The listing builds one solid part. Answer for the finished solid, in the listing's coordinates (mm). A direction names the side the tool comes from. Coordinates: 2 decimals unless noted, no trailing zeros. Write each loop counter-clockwise with the first axis right and the second up, starting at its lowest first coordinate (ties: lowest second). Pieces come first, ordered by that corner, then holes. Notation, with made-up numbers: M 53,53 L 81,53 A36 cw 81,92 Z; hole C 32.25,56 d1. An arc over 180 degrees is marked long. Answer as CSV lines item,"result".
```python
from build123d import *

# Parameters (mm, degrees)
SKETCH1_R           = 37.5
BOSS_EXTRUDE1_DEPTH = 10
BOSS_EXTRUDE2_START = 10
BOSS_EXTRUDE2_DEPTH = 10
SKETCH3_R           = 2.55
CUT_EXTRUDE1_DEPTH  = 10


with BuildPart() as part:
    # Sketch1 → Boss-Extrude1 (new body)
    with BuildSketch(Plane(origin=(0, 0, 0), x_dir=(1, 0, 0), z_dir=(0, 1, 0))):
        with Locations(Location((11.945516858, 0, 0), (0, 0, 270))):
            Circle(SKETCH1_R)
    extrude(amount=BOSS_EXTRUDE1_DEPTH)

    # Sketch2 → Boss-Extrude2 (add)
    with BuildSketch(Plane(origin=(0, 0, 0), x_dir=(1, 0, 0), z_dir=(0, 1, 0)).offset(BOSS_EXTRUDE2_START)):
        with BuildLine():
            Line((-6.304483142, 19.484324941), (30.195516858, 19.484324941))
            ThreePointArc((30.195516858, 19.484324941), (37.26658467, 16.555392753), (40.195516858, 9.484324941))
            Line((40.195516858, 9.484324941), (40.195516858, -9.205373472))
            ThreePointArc((40.195516858, -9.205373472), (37.270385296, -16.272638614), (30.20626954, -19.205367691))
            Line((30.20626954, -19.205367691), (-6.29373046, -19.244615001))
            ThreePointArc((-6.29373046, -19.244615001), (-13.371748284, -16.319489219), (-16.304483142, -9.244620782))
            Line((-16.304483142, -9.244620782), (-16.304483142, 9.484324941))
            ThreePointArc((-16.304483142, 9.484324941), (-13.375550954, 16.555392753), (-6.304483142, 19.484324941))
        make_face()
        Polygon((-11.304483142, -14.250000016), (35.195516858, -14.200000018), (35.195516858, 14.484324941), (-11.304483142, 14.484324941), align=None, mode=Mode.SUBTRACT)
    extrude(amount=BOSS_EXTRUDE2_DEPTH)

    # Sketch3 → Cut-Extrude1 (cut)
    with BuildSketch(Plane(origin=(0, 10, 0), x_dir=(1, 0, 0), z_dir=(0, 1, 0))):
        with Locations(Location((-21.054483142, -5, 0), (0, 0, 270))):
            Circle(SKETCH3_R)
        with Locations(Location((-21.054483142, 5, 0), (0, 0, 90))):
            Circle(SKETCH3_R)
        with Locations(Location((44.945516858, -5, 0), (0, 0, 90))):
            Circle(SKETCH3_R)
        with Locations(Location((44.945516858, 5, 0), (0, 0, 270))):
            Circle(SKETCH3_R)
    extrude(amount=-CUT_EXTRUDE1_DEPTH, mode=Mode.SUBTRACT)


solid = part.part
```
Q1. For faces 5 (the flat face through (-11.304, 15, 0)), 6 (the cylindrical face through (-13.45, 14.93, -16.48)), 7 (the cylindrical face through (37.19, 14.93, -16.63)), determine the directions among +Z, -Z, +X, -X, +Y, -Y from which every point of the face is accessible in a straight line to the end or side of a thin tool.
Output:
face 5,"+Y"
face 6,"-Z, -X, +Y"
face 7,"-Z, +X, +Y"
Q2. Find section B-B (z = -5). Give the vertices of the cut face in (x, y).
Output:
outline,"M -25.22,0 L -23.6,0 L -23.6,10 L -25.22,10 Z; M -18.5,0 L 42.4,0 L 42.4,10 L 40.2,10 L 40.2,20 L 35.2,20 L 35.2,10 L -11.3,10 L -11.3,20 L -16.3,20 L -16.3,10 L -18.5,10 Z; M 47.5,0 L 49.11,0 L 49.11,10 L 47.5,10 Z"
Q3. Find section D-D (x = 16). Give the vertices of the cut face in (y, z), and give its area (3 significant figures).
Output:
outline,"M 0,-37.28 L 10,-37.28 L 10,-19.48 L 20,-19.48 L 20,-14.48 L 10,-14.48 L 10,14.22 L 20,14.22 L 20,19.22 L 10,19.22 L 10,37.28 L 0,37.28 Z"
area,"846 mm2"
Q4. Straight lines are drawn through the part: line 1 (Z direction, x = -21.5, y = 2.75); line 2 (X direction, y = 4.25, z = -5); line 3 (Z direction, x = 2, y = 10.75). For each, find the intervals that lie inside material, in ascending order.
Output:
line 1,"-16.96 to -7.51, -2.49 to 2.49, 7.51 to 16.96"
line 2,"-25.22 to -23.6, -18.5 to 42.4, 47.5 to 49.11"
line 3,"-19.48 to -14.48, 14.24 to 19.24"
Q5. Find section C-C (x = 24). Give the vertices of the cut face in (y, z).
Output:
outline,"M 0,-35.51 L 10,-35.51 L 10,-19.48 L 20,-19.48 L 20,-14.48 L 10,-14.48 L 10,14.21 L 20,14.21 L 20,19.21 L 10,19.21 L 10,35.51 L 0,35.51 Z"
Q6. Flat-ended cylindrical pins translate along their axes: pin 1 Ø8.5 at (x, z) = (6, 0.5) entering from +Y; pin 2 Ø3 at (y, z) = (13, -4.5) entering from +X; pin 3 Ø4 at (x, y) = (-4, 16.5) entering from -Z. Find the tip coordinate at first contact, or state that the pin passes through.
Output:
pin 1,"y = 10"
pin 2,"x = 40.2"
pin 3,"z = -19.48"
Q7. Find section A-A (y = 12.75). Give the vertices of the cut face in (x, z), and give its area (3 significant figures).
Output:
outline,"M -16.3,-9.48 A10 ccw -6.3,-19.48 L 30.2,-19.48 A10 ccw 40.2,-9.48 L 40.2,9.21 A10 ccw 30.21,19.21 L -6.29,19.24 A10 ccw -16.3,9.24 Z; hole M -11.3,-14.48 L 35.2,-14.48 L 35.2,14.2 L -11.3,14.25 Z"
area,"766 mm2"
Q8. The mould has two halves that part along X. Classify faces 1 (the flat face through (12, 10, 0)), 2 (the flat face through (-16.304, 15, 0)), 3 (the cylindrical face through (-21.82, 5.07, -7.432)), 4 (the flat face through (12, 15, -19.484)): pulls with the +X half, pulls with the -X half, needs draft (parallel to the pull), parting line crosses it, or undercut.
Output:
face 1,"undercut"
face 2,"pulls with the -X half"
face 3,"undercut"
face 4,"needs draft"
